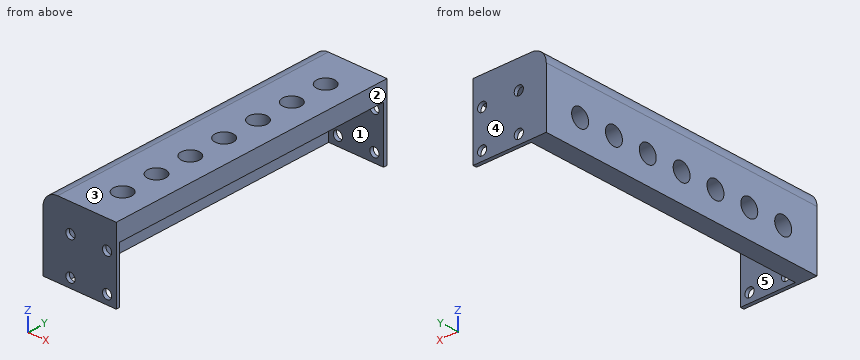
```python
from build123d import *

# Parameters (mm, degrees)
BOSS_EXTRUDE1_DEPTH = 203.2
FILLET1_R           = 10.16
SKETCH3_R           = 6.35
CUT_EXTRUDE1_DEPTH  = 51.8
SKETCH4_R           = 6.35
CUT_EXTRUDE2_DEPTH  = 51.8
SKETCH5_R           = 3.175
BOSS_EXTRUDE2_DEPTH = 2.54


with BuildPart() as part:
    # Sketch2 → Boss-Extrude1 (new body)
    with BuildSketch(Plane(origin=(0, 0, 0), x_dir=(1, 0, 0), z_dir=(0, 1, 0))):
        Polygon((0, 0), (50.8, 0), (50.8, 12.7), (12.7, 12.7), (12.7, 50.8), (0, 50.8), align=None)
    extrude(amount=BOSS_EXTRUDE1_DEPTH)

    # Fillet1
    fillet1_edges = [part.edges().sort_by_distance(p)[0] for p in [
        (12.7, 101.6, -12.7),
        (0, 101.6, 0),
    ]]
    fillet(fillet1_edges, radius=FILLET1_R)

    # Sketch3 → Cut-Extrude1 (cut, through all)
    with BuildSketch(Plane.XY):
        with Locations((31.75, 177.8)):
            Circle(SKETCH3_R)
        with Locations((31.75, 152.4)):
            Circle(SKETCH3_R)
        with Locations((31.75, 127)):
            Circle(SKETCH3_R)
        with Locations((31.75, 101.6)):
            Circle(SKETCH3_R)
        with Locations((31.75, 76.2)):
            Circle(SKETCH3_R)
        with Locations((31.75, 50.8)):
            Circle(SKETCH3_R)
        with Locations((31.75, 25.4)):
            Circle(SKETCH3_R)
    extrude(amount=-CUT_EXTRUDE1_DEPTH, mode=Mode.SUBTRACT)

    # Sketch4 → Cut-Extrude2 (cut, through all)
    with BuildSketch(Plane.ZY):
        with Locations((-31.75, 177.8)):
            Circle(SKETCH4_R)
        with Locations((-31.75, 152.4)):
            Circle(SKETCH4_R)
        with Locations((-31.75, 127)):
            Circle(SKETCH4_R)
        with Locations((-31.75, 101.6)):
            Circle(SKETCH4_R)
        with Locations((-31.75, 76.2)):
            Circle(SKETCH4_R)
        with Locations((-31.75, 50.8)):
            Circle(SKETCH4_R)
        with Locations((-31.75, 25.4)):
            Circle(SKETCH4_R)
    extrude(amount=-CUT_EXTRUDE2_DEPTH, mode=Mode.SUBTRACT)

    # Sketch5 → Boss-Extrude2 (add)
    with BuildSketch(Plane(origin=(0, 203.2, 0), x_dir=(1, 0, 0), z_dir=(0, 1, 0))):
        with BuildLine():
            Line((50.8, 50.8), (12.7, 50.8))
            Line((12.7, 50.8), (12.7, 22.86))
            ThreePointArc((12.7, 22.86), (15.675795103, 15.675795103), (22.86, 12.7))
            Line((22.86, 12.7), (50.8, 12.7))
            Line((50.8, 12.7), (50.8, 50.8))
        make_face()
        with Locations((19.05, 19.05)):
            Circle(SKETCH5_R, mode=Mode.SUBTRACT)
        with Locations((44.45, 19.05)):
            Circle(SKETCH5_R, mode=Mode.SUBTRACT)
        with Locations((19.05, 44.45)):
            Circle(SKETCH5_R, mode=Mode.SUBTRACT)
        with Locations((44.45, 44.45)):
            Circle(SKETCH5_R, mode=Mode.SUBTRACT)
    boss_extrude2 = extrude(amount=-BOSS_EXTRUDE2_DEPTH)

    # Mirror1: Boss-Extrude2 across plane
    add(boss_extrude2.mirror(Plane.ZX.offset(101.6)))


solid = part.part
```
Geometry check sheet. Reference: the model listing, model coordinates, mm. Face numbers are marked on the shaded views. A direction names the side the tool comes from. Coordinates: 2 decimals unless noted, no trailing zeros. Order: outer loops, then holes, each group sorted by start corner. A loop starts at its lowest first (then second) coordinate and runs counter-clockwise, first axis right, second up. Notation, with made-up numbers: (-15.75, -14) - (43.25, -14) arc R23 ccw to (43.25, 10) - close; hole circle Ø2 at (63.25, 71). An arc over 180 degrees is marked (long way). Answer in a Markdown table with one row per item. Add a question column.
1. Section check A-A (z = -44.45). Enter the section's corners in (x, y) (3 decimals).
2. Gauge pin test, flat ends, axial feed: pin 1 Ø5.5 at (x, z) = (19.05, -19.05) entering from +Y; pin 2 Ø6 at (x, y) = (36, 100.5) entering from -Z; pin 3 Ø10 at (y, z) = (59.5, -20) entering from +X; pin 4 Ø2 at (y, z) = (75, -25.5) entering from +X. Record the tip position at first contact, or that the pin passes through.
3. Access from +Z, -Z, +X, -X, +Y, -Y to the whole of each face (thin tool, end or side, straight path). Record for the marked faces 1 and 2.
4. Section check B-B (y = 101.6). Enter the section's corners in (x, z), plus the area to 3 significant figures.
5. Draft check along Y on the marked faces 3, 4 and 5. Enter one of: +Y half, -Y half, draft (parallel to the pull), parting line (faces both ways), or undercut.
6. Material ranges on L1, parallel to X at y = 201.4, z = -44.45 (3 decimals); L2, parallel to Z at x = 44, y = 202; L3, parallel to Z at x = 9.5, y = 51, recorded low to high. Write a range as [from, to].
7. Section check D-D (y = 62). Enter the section's corners in (x, z), plus the area to 3 significant figures.
8. Section check C-C (x = 19.05). Enter the section's corners in (y, z) (3 decimals), plus the area to 3 significant figures.
Data:
| question | item | result |
|---|---|---|
| 1 | outline | (0, 0) - (15.875, 0) - (15.875, 2.54) - (12.7, 2.54) - (12.7, 200.66) - (15.875, 200.66) - (15.875, 203.2) - (0, 203.2) - close; (22.225, 0) - (41.275, 0) - (41.275, 2.54) - (22.225, 2.54) - close; (22.225, 200.66) - (41.275, 200.66) - (41.275, 203.2) - (22.225, 203.2) - close; (47.625, 0) - (50.8, 0) - (50.8, 2.54) - (47.625, 2.54) - close; (47.625, 200.66) - (50.8, 200.66) - (50.8, 203.2) - (47.625, 203.2) - close |
| 2 | pin 1 | passes through |
| 2 | pin 2 | stops at z = -12.7 |
| 2 | pin 3 | stops at x = 16.42 |
| 2 | pin 4 | stops at x = 12.7 |
| 3 | face 1 | -Z, +X |
| 3 | face 2 | +Z, -Z, +X, +Y, -Y |
| 4 | outline | (0, -50.8) - (12.7, -50.8) - (12.7, -38.1) - (0, -38.1) - close; (0, -25.4) - (12.7, -25.4) - (12.7, -22.86) arc R10.16 cw to (22.86, -12.7) - (25.4, -12.7) - (25.4, 0) - (10.16, 0) arc R10.16 ccw to (0, -10.16) - close; (38.1, -12.7) - (50.8, -12.7) - (50.8, 0) - (38.1, 0) - close |
| 4 | area | 806 mm² |
| 5 | face 3 | draft |
| 5 | face 4 | +Y half |
| 5 | face 5 | undercut |
| 6 | L1 | x = [0, 15.875], [22.225, 41.275], [47.625, 50.8] |
| 6 | L2 | z = [-50.8, -47.59], [-41.31, -22.19], [-15.91, 0] |
| 6 | L3 | z = [-50.8, -38.1], [-25.4, -0.02] |
| 7 | outline | (0, -50.8) - (12.7, -50.8) - (12.7, -22.86) arc R10.16 cw to (22.86, -12.7) - (50.8, -12.7) - (50.8, 0) - (10.16, 0) arc R10.16 ccw to (0, -10.16) - close |
| 7 | area | 1,130 mm² |
| 8 | outline | (0, -50.8) - (2.54, -50.8) - (2.54, -47.625) - (0, -47.625) - close; (0, -41.275) - (2.54, -41.275) - (2.54, -22.225) - (0, -22.225) - close; (0, -15.875) - (2.54, -15.875) - (2.54, -13.441) - (200.66, -13.441) - (200.66, -15.875) - (203.2, -15.875) - (203.2, 0) - (0, 0) - close; (200.66, -50.8) - (203.2, -50.8) - (203.2, -47.625) - (200.66, -47.625) - close; (200.66, -41.275) - (203.2, -41.275) - (203.2, -22.225) - (200.66, -22.225) - close |
| 8 | area | 2,860 mm² |
